```python
from build123d import *

# Parameters (mm, degrees)
HEX_HEAD_DEPTH     = 3
SKETCH2_R          = 1.75
CUT_EXTRUDE1_DEPTH = 3


with BuildPart() as part:
    # Sketch1 → Hex_Head (new body)
    with BuildSketch(Plane(origin=(0, 0, 0), x_dir=(0, 0, -1), z_dir=(1, 0, 0))):
        Polygon((3.5, -2.020725942), (3.5, 2.020725942), (0, 4.041451884), (-3.5, 2.020725942), (-3.5, -2.020725942), (0, -4.041451884), align=None)
    extrude(amount=HEX_HEAD_DEPTH)

    # Sketch2 → Cut-Extrude1 (cut)
    with BuildSketch(Plane.ZY):
        Circle(SKETCH2_R)
    extrude(amount=-CUT_EXTRUDE1_DEPTH, mode=Mode.SUBTRACT)


solid = part.part
```
Here's how the part is built. I have some questions about the finished solid (model axes, mm). Round coordinates to 2 decimals unless told otherwise and drop trailing zeros. Order: outer loops, then holes, each group sorted by start corner. A loop starts at its lowest first (then second) coordinate and runs counter-clockwise, first axis right, second up. Notation, with made-up numbers: (66, 84.25) -> (82, 84.25) arc R25 cw to (82, 106.25) -> close; hole circle Ø8 at (18, 22). An arc over 180 degrees is marked (long way). Use a Markdown table: item, result. Add a question column.
(1) I need wall thicknesses on line 1 along Y through (x, z) = (0.8, -1.25); line 2 along Z through (x, y) = (2, 1); line 3 along Z through (x, y) = (2.25, 0.5). Which ranges of each line are inside material? Lowest first, please.
(2) Suppose I cut it at C-C, the plane z = -1. Please give me the cut outline in (x, y), and give its area (3 significant figures).
(3) Suppose I cut it at D-D, the plane z = -2. Please give me the cut outline in (x, y), and give its area (3 significant figures).
(4) For pin 1 Ø2 at (y, z) = (0, 0) entering from -X, with a flat end and sliding along its axis, tell me the tip position at first contact or that it passes through.
(5) Suppose I cut it at A-A, the plane y = 0. Please give me the cut outline in (x, z), and give its area (3 significant figures).
(6) If we mould it in two halves opening along X, with no side actions, what happens to faces 1 (the face through (0, -1, 2)), 2 (the face through (1.479, -3.045, -1.726)), 3 (the face through (3, -1, 2))? For each: released by +X, released by -X, zero draft, split by the parting line, or undercut.
(7) Suppose I cut it at B-B, the plane x = 1.2. Please give me the cut outline in (y, z), and give its area (3 significant figures).
Verdict:
| question | item | result |
|---|---|---|
| 1 | line 1 | -3.32 to -1.22, 1.22 to 3.32 |
| 1 | line 2 | -3.5 to -1.44, 1.44 to 3.5 |
| 1 | line 3 | -3.5 to -1.68, 1.68 to 3.5 |
| 2 | outline | (0, -3.46) -> (3, -3.46) -> (3, -1.44) -> (0, -1.44) -> close; (0, 1.44) -> (3, 1.44) -> (3, 3.46) -> (0, 3.46) -> close |
| 2 | area | 12.2 mm2 |
| 3 | outline | (0, -2.89) -> (3, -2.89) -> (3, 2.89) -> (0, 2.89) -> close |
| 3 | area | 17.3 mm2 |
| 4 | pin 1 | through |
| 5 | outline | (0, -3.5) -> (3, -3.5) -> (3, -1.75) -> (0, -1.75) -> close; (0, 1.75) -> (3, 1.75) -> (3, 3.5) -> (0, 3.5) -> close |
| 5 | area | 10.5 mm2 |
| 6 | face 1 | released by -X |
| 6 | face 2 | zero draft |
| 6 | face 3 | released by +X |
| 7 | outline | (-4.04, 0) -> (-2.02, -3.5) -> (2.02, -3.5) -> (4.04, 0) -> (2.02, 3.5) -> (-2.02, 3.5) -> close; hole circle Ø3.5 at (0, 0) |
| 7 | area | 32.8 mm2 |
